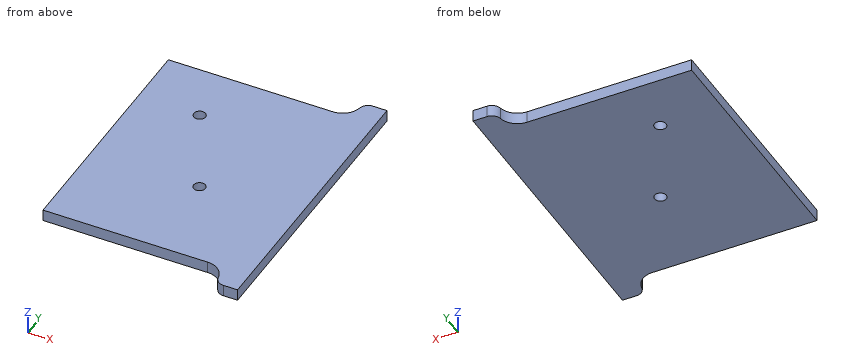
from build123d import *

# Parameters (mm, degrees)
F0_W     = 6.35
F0_H     = 6.35
F1_DEPTH = 3.175
F0_R     = 1.5875
F2_DEPTH = 3.175
F3_R     = 2.54
F4_R     = 5.08


with BuildPart() as f1:
    # F0 (on Top) → F1 (new body)
    with BuildSketch(Plane.XY):
        Polygon((60.1484737206, 7.2537393374), (10.6184737206, 7.2537393374), (10.6184737206, -58.7862606626), (60.1484737206, -58.7862606626), (66.4984737206, -58.7862606626), (66.4984737206, 7.2537393374), align=None)
        with BuildLine():
            ThreePointArc((22.7113279829, -20.4435077931), (20.0093369897, 1.8826225402), (39.9210240364, -8.5711600259))
            ThreePointArc((39.9210240364, -8.5711600259), (39.8123227124, -10.2292304863), (39.4880795243, -11.8589175682))
            ThreePointArc((39.4880795243, -11.8589175682), (55.0511803081, -18.0157023959), (61.5383527356, -33.4440107709))
            ThreePointArc((61.5383527356, -33.4440107709), (33.0934006719, -53.9168643142), (22.7113279829, -20.4435077931))
        make_face(mode=Mode.SUBTRACT)
        with Locations((63.3234737206, 10.4287393374)):
            Rectangle(F0_W, F0_H)
        with Locations((63.3234737206, -61.9612606626)):
            Rectangle(F0_W, F0_H)
    extrude(amount=F1_DEPTH)

    # F0 (on Top) → F2 (join)
    with BuildSketch(Plane.XY):
        Polygon((60.1484737206, 7.2537393374), (10.6184737206, 7.2537393374), (10.6184737206, -58.7862606626), (60.1484737206, -58.7862606626), (66.4984737206, -58.7862606626), (66.4984737206, 7.2537393374), align=None)
        with BuildLine():
            ThreePointArc((22.7113279829, -20.4435077931), (20.0093369897, 1.8826225402), (39.9210240364, -8.5711600259))
            ThreePointArc((39.9210240364, -8.5711600259), (39.8123227124, -10.2292304863), (39.4880795243, -11.8589175682))
            ThreePointArc((39.4880795243, -11.8589175682), (55.0511803081, -18.0157023959), (61.5383527356, -33.4440107709))
            ThreePointArc((61.5383527356, -33.4440107709), (33.0934006719, -53.9168643142), (22.7113279829, -20.4435077931))
        make_face(mode=Mode.SUBTRACT)
        with BuildLine():
            ThreePointArc((39.4880795243, -11.8589175682), (39.8123227124, -10.2292304863), (39.9210240364, -8.5711600259))
            ThreePointArc((39.9210240364, -8.5711600259), (20.0093369897, 1.8826225402), (22.7113279829, -20.4435077931))
            ThreePointArc((22.7113279829, -20.4435077931), (26.0598460264, -16.9141141774), (30.1135988267, -14.2240806058))
            ThreePointArc((30.1135988267, -14.2240806058), (34.6667436153, -12.5100024328), (39.4880795243, -11.8589175682))
        make_face()
        with BuildLine():
            ThreePointArc((33.5710240364, -8.5711600259), (32.6381427317, -11.8843646741), (30.1135988267, -14.2240806058))
            ThreePointArc((30.1135988267, -14.2240806058), (21.8039053411, -5.2579553777), (33.5710240364, -8.5711600259))
        make_face(mode=Mode.SUBTRACT)
        with BuildLine():
            ThreePointArc((30.1135988267, -14.2240806058), (26.0598460264, -16.9141141774), (22.7113279829, -20.4435077931))
            ThreePointArc((22.7113279829, -20.4435077931), (33.0061734451, -19.8770012736), (39.4880795243, -11.8589175682))
            ThreePointArc((39.4880795243, -11.8589175682), (34.6667436153, -12.5100024328), (30.1135988267, -14.2240806058))
        make_face()
        with BuildLine():
            ThreePointArc((39.4880795243, -11.8589175682), (33.0061734451, -19.8770012736), (22.7113279829, -20.4435077931))
            ThreePointArc((22.7113279829, -20.4435077931), (33.0934006719, -53.9168643142), (61.5383527356, -33.4440107709))
            ThreePointArc((61.5383527356, -33.4440107709), (55.0511803081, -18.0157023959), (39.4880795243, -11.8589175682))
        make_face()
        with Locations((39.9483527356, -33.4440107709)):
            Circle(F0_R, mode=Mode.SUBTRACT)
        with BuildLine():
            ThreePointArc((33.5710240364, -8.5711600259), (21.8039053411, -5.2579553777), (30.1135988267, -14.2240806058))
            ThreePointArc((30.1135988267, -14.2240806058), (32.6381427317, -11.8843646741), (33.5710240364, -8.5711600259))
        make_face()
        with Locations((27.2210240364, -8.5711600259)):
            Circle(F0_R, mode=Mode.SUBTRACT)
    extrude(amount=F2_DEPTH)

    # F3
    f3_edges = [f1.edges().sort_by_distance(p)[0] for p in [
        (60.148474, -65.136261, 1.5875),
        (60.148474, 13.603739, 1.5875),
    ]]
    fillet(f3_edges, radius=F3_R)

    # F4
    f4_edges = [f1.edges().sort_by_distance(p)[0] for p in [
        (60.148474, -58.786261, 1.5875),
        (60.148474, 7.253739, 1.5875),
    ]]
    fillet(f4_edges, radius=F4_R)


solid = f1.part
Read the model definition and answer for the solid it produces. Units are mm, in the model's axes. Round coordinates to 2 decimals unless told otherwise and drop trailing zeros. Write each loop counter-clockwise with the first axis right and the second up, starting at its lowest first coordinate (ties: lowest second). Pieces come first, ordered by that corner, then holes.
Q1. Find section B-B on z = 1.3. State how many separate pieces and enclosed holes the cut face has, and give its area (3 significant figures).
Values:
separate pieces: 1
enclosed holes: 2
area: 3,760 mm2
Q2. Find section A-A on x = 44.5. Determine the outline of the cut face in (y, z) (3 decimals), and give its area (3 significant figures).
Values:
outline: (-58.786, 0) - (7.254, 0) - (7.254, 3.175) - (-58.786, 3.175) - close
area: 210 mm2
Q3. Flat-ended cylindrical pins translate along their axes: P1, Ø1, axis at x = 26, z = 0.5, coming from the +Y side; P2, Ø3.5, axis at x = 27.22, y = -8.57, coming from the -Z side; P3, Ø1.6, axis at x = 42.5, z = 2.5, coming from the -Y side; P4, Ø1.5, axis at x = 58.5, z = 2.5, coming from the +Y side. Find the tip coordinate at first contact, or state that the pin passes through.
Values:
P1: stops at y = 7.25
P2: stops at z = 0
P3: stops at y = -58.79
P4: stops at y = 9.3
Q4. Straight lines are drawn through the part: line 1 (Y direction, x = 35.5, z = 2.45); line 2 (Y direction, x = 28, z = 2.45); line 3 (Y direction, x = 39.5, z = 2.1). For each, find the intervals that lie inside material, in ascending order.
Values:
line 1: y = -58.79 to 7.25
line 2: y = -58.79 to -9.95, -7.19 to 7.25
line 3: y = -58.79 to -34.97, -31.92 to 7.25
